For this review, take the finished solid that the model builds, in its own axes (mm). A direction names the side the tool comes from. Coordinates: 2 decimals unless noted, no trailing zeros. Write each loop counter-clockwise with the first axis right and the second up, starting at its lowest first coordinate (ties: lowest second). Pieces come first, ordered by that corner, then holes. Notation, with made-up numbers: M -30.5,-38.75 L -12.5,-38.75 A15 ccw -12.5,-9.75 Z; hole C 28.25,-13 d6. An arc over 180 degrees is marked long. One line per question, with ' | ' between items.
from build123d import *

# Parameters (mm, degrees)
CROQUIS1_R              = 20
CROQUIS1_R_2            = 2.5
CROQUIS1_R_3            = 1.5
SALIENTE_EXTRUIR1_DEPTH = 5
CORTAR_EXTRUIR1_DEPTH   = 29.722813233
MATRIZC1_COUNT          = 18
CROQUIS3_R              = 3.7
CORTAR_EXTRUIR2_DEPTH   = 2.5
CROQUIS4_R              = 2.25
CORTAR_EXTRUIR3_DEPTH   = 2.5


with BuildPart() as part:
    # Croquis1 → Saliente-Extruir1 (new body)
    with BuildSketch(Plane.XY):
        Circle(CROQUIS1_R)
        Circle(CROQUIS1_R_2, mode=Mode.SUBTRACT)
        with Locations((0, 6)):
            Circle(CROQUIS1_R_3, mode=Mode.SUBTRACT)
    extrude(amount=SALIENTE_EXTRUIR1_DEPTH)

    # Croquis2 → Cortar-Extruir1 (cut, through all)
    with BuildSketch(Plane.XY.offset(5)):
        with BuildLine():
            ThreePointArc((2.678584333, 19.819818011), (0, 20), (-2.678584333, 19.819818011))
            ThreePointArc((-2.678584333, 19.819818011), (-1.82600889, 18.733131722), (-1.522223543, 17.385731841))
            ThreePointArc((-1.522223543, 17.385731841), (-1.19593308, 16.445057276), (-0.5915417, 15.653827117))
            ThreePointArc((-0.5915417, 15.653827117), (0, 15.665), (0.5915417, 15.653827117))
            ThreePointArc((0.5915417, 15.653827117), (1.19593308, 16.445057276), (1.522223543, 17.385731841))
            ThreePointArc((1.522223543, 17.385731841), (1.82600889, 18.733131722), (2.678584333, 19.819818011))
        make_face()
    cortar_extruir1 = extrude(amount=-CORTAR_EXTRUIR1_DEPTH, mode=Mode.SUBTRACT)

    # MatrizC1: Cortar-Extruir1 ×18 about axis
    matrizc1_axis = Axis((0, 0, 0), (0, 0, 1))
    for i in range(1, MATRIZC1_COUNT):
        add(cortar_extruir1.rotate(matrizc1_axis, i * 360 / MATRIZC1_COUNT), mode=Mode.SUBTRACT)

    # Croquis3 → Cortar-Extruir2 (cut)
    with BuildSketch(Plane.XY.offset(5)):
        Circle(CROQUIS3_R)
    extrude(amount=-CORTAR_EXTRUIR2_DEPTH, mode=Mode.SUBTRACT)

    # Croquis4 → Cortar-Extruir3 (cut)
    with BuildSketch(Plane(origin=(0, 0, 0), x_dir=(-1, 0, 0), z_dir=(0, 0, -1))):
        with Locations((0, 6)):
            Circle(CROQUIS4_R)
    extrude(amount=-CORTAR_EXTRUIR3_DEPTH, mode=Mode.SUBTRACT)


solid = part.part
1. Machinability: for faces 1 (the cylindrical face through (13.423, 13.169, 2.535)), 2 (the cylindrical face through (15.3, -10.93, 2.54)), 3 (the cylindrical face through (-13.56, -7.84, 2.54)), which of the approach directions +Z, -Z, +X, -X, +Y, -Y give a long, thin tool a straight path to every point of the face, cutting with its end or side? Answer none if there is none.
Computed values:
face 1: +Z, -Z, +Y | face 2: +Z, -Z, +X | face 3: +Z, -Z
2. For line 1 along X through (y, z) = (0, 0.75); line 2 along Y through (x, z) = (0, 1.6) (3 decimals); line 3 along Y through (x, z) = (0.5, 4.2), list the stretches that pass through material, from the lowest coordinate up.
Computed values:
line 1: x = -20 to -2.5, 2.5 to 20 | line 2: y = -15.665 to -2.5, 2.5 to 3.75, 8.25 to 15.665 | line 3: y = -15.66 to -3.67, 3.67 to 4.59, 7.41 to 15.66
3. Take a section at D-D on z = 4. Give the number of separate pieces and of enclosed holes in the cut face, plus the area to 3 significant figures.
Computed values:
separate pieces: 1 | enclosed holes: 2 | area: 958 mm2
4. Take a section at C-C on y = -13. State the section outline as (x, z) points.
Computed values:
outline: M -15.2,0 L -13.11,0 L -13.11,5 L -15.2,5 Z; M -9.6,0 L 9.6,0 L 9.6,5 L -9.6,5 Z; M 13.11,0 L 15.2,0 L 15.2,5 L 13.11,5 Z
5. Take a section at A-A on x = 0. State the section outline as (y, z) points (3 decimals), plus the area to 3 significant figures.
Computed values:
outline: M -15.665,0 L -2.5,0 L -2.5,2.5 L -3.7,2.5 L -3.7,5 L -15.665,5 Z; M 2.5,0 L 3.75,0 L 3.75,2.5 L 4.5,2.5 L 4.5,5 L 3.7,5 L 3.7,2.5 L 2.5,2.5 Z; M 7.5,2.5 L 8.25,2.5 L 8.25,0 L 15.665,0 L 15.665,5 L 7.5,5 Z | area: 107 mm2
6. Draft analysis for pull direction X (two halves, no side actions). For faces 4 (the cylindrical face through (18.79, -6.85, 2.46)), 5 (the cylindrical face through (-11.474, -11.824, 2.535)), 6 (the cylindrical face through (-13.65, -9.27, 2.54)), state which applies: pulls with the +X half, pulls with the -X half, needs draft (parallel to the pull), parting line crosses it, or undercut.
Computed values:
face 4: pulls with the +X half | face 5: undercut | face 6: pulls with the -X half
7. Clearance check with flat-ended pins moving along their axes: P1, Ø4.5, axis at x = 0, y = 0, coming from the -Z side; P2, Ø3.5, axis at x = 0.5, y = -1.5, coming from the +Z side. State where each tip first meets the part, or that it passes through.
Computed values:
P1: passes through | P2: stops at z = 2.5
8. Take a section at B-B on y = 0. State the section outline as (x, z) points, plus the area to 3 significant figures.
Computed values:
outline: M -20,0 L -2.5,0 L -2.5,2.5 L -3.7,2.5 L -3.7,5 L -20,5 Z; M 2.5,0 L 20,0 L 20,5 L 3.7,5 L 3.7,2.5 L 2.5,2.5 Z | area: 169 mm2
